```python
from build123d import *

# Parameters (mm, degrees)
SKETCH1_W            = 16.31
SKETCH1_H            = 16.31
SKETCH1_R            = 4.5
BOSS_EXTRUDE1_DEPTH  = 4
SKETCH3_R            = 1.5
CUT_EXTRUDE1_DEPTH   = 4
BOSS_EXTRUDE2_DEPTH  = 4
BOSS_EXTRUDE6_DEPTH  = 4
CUT_EXTRUDE3_DEPTH   = 4
BOSS_EXTRUDE7_DEPTH  = 4
BOSS_EXTRUDE9_DEPTH  = 4
SKETCH17_OUTSIDE_W   = 136.165
SKETCH17_OUTSIDE_H   = 117.232
CUT_EXTRUDE4_DEPTH   = 4
SKETCH18_R           = 1.5
BOSS_EXTRUDE10_DEPTH = 4
CUT_EXTRUDE5_DEPTH   = 4
SKETCH20_R           = 2
CUT_EXTRUDE6_DEPTH   = 10
SKETCH21_R           = 3
CUT_EXTRUDE7_DEPTH   = 2


with BuildPart() as part:
    # Sketch1 → Boss-Extrude1 (new body)
    with BuildSketch(Plane(origin=(0, 0, 0), x_dir=(1, 0, 0), z_dir=(0, 1, 0))):
        Rectangle(SKETCH1_W, SKETCH1_H)
        with Locations(Location((0, 0, 0), (0, 0, 270))):
            Circle(SKETCH1_R, mode=Mode.SUBTRACT)
    extrude(amount=BOSS_EXTRUDE1_DEPTH)

    # Sketch3 → Cut-Extrude1 (cut)
    with BuildSketch(Plane(origin=(0, 4, 0), x_dir=(1, 0, 0), z_dir=(0, 1, 0))):
        with Locations(Location((5.656854249, 5.656854249, 0), (0, 0, 270))):
            Circle(SKETCH3_R)
        with Locations(Location((5.656854249, -5.656854249, 0), (0, 0, 270))):
            Circle(SKETCH3_R)
        with Locations(Location((-5.656854249, -5.656854249, 0), (0, 0, 270))):
            Circle(SKETCH3_R)
        with Locations(Location((-5.656854249, 5.656854249, 0), (0, 0, 270))):
            Circle(SKETCH3_R)
    extrude(amount=-CUT_EXTRUDE1_DEPTH, mode=Mode.SUBTRACT)

    # Sketch4 → Boss-Extrude2 (add)
    with BuildSketch(Plane(origin=(0, 4, 0), x_dir=(1, 0, 0), z_dir=(0, 1, 0))):
        Polygon((8.155, -8.155), (0, -8.155), (0, -10.655), (10.655, -10.655), (10.655, 0), (8.155, 0), align=None)
    extrude(amount=-BOSS_EXTRUDE2_DEPTH)

    # Sketch9 → Boss-Extrude6 (add)
    with BuildSketch(Plane(origin=(0, 4, 0), x_dir=(1, 0, 0), z_dir=(0, 1, 0))):
        Polygon((71.061407011, -58.982568069), (7.593139788, -10.281653748), (10.613791504, -4.032054751), (84.193483815, -43.982568069), (90.501950314, -50.291034568), (96.061407011, -50.291034568), (96.061407011, -73.982568069), (81.061407011, -73.982568069), (81.061407011, -68.982568069), align=None)
    extrude(amount=-BOSS_EXTRUDE6_DEPTH)

    # Sketch12 → Cut-Extrude3 (cut)
    with BuildSketch(Plane(origin=(0, 4, 0), x_dir=(1, 0, 0), z_dir=(0, 1, 0))):
        Polygon((87.278639473, -47.258318902), (85.780514725, -48.583317861), (89.960889469, -52.761034568), (90.501950314, -52.761034568), (96.061407011, -52.761034568), (96.061407011, -50.291034568), (90.501950314, -50.291034568), (87.347717064, -47.136801318), align=None)
    extrude(amount=-CUT_EXTRUDE3_DEPTH, mode=Mode.SUBTRACT)

    # Sketch13 → Boss-Extrude7 (add)
    with BuildSketch(Plane(origin=(0, 4, 0), x_dir=(1, 0, 0), z_dir=(0, 1, 0))):
        Polygon((81.061407011, -73.982568069), (81.061407011, -77.282568069), (96.561407011, -77.282568069), (96.561407011, -52.761034568), (96.061407011, -52.761034568), (96.061407011, -73.982568069), align=None)
    extrude(amount=-BOSS_EXTRUDE7_DEPTH)

    # Sketch16 → Boss-Extrude9 (add)
    with BuildSketch(Plane(origin=(0, 4, 0), x_dir=(1, 0, 0), z_dir=(0, 1, 0))):
        Polygon((0, -10.655), (-10, -10.655), (-10, 10.345), (10.655, 10.345), (10.655, 0), (8.155, 0), (8.155, 8.155), (-8.155, 8.155), (-8.155, -8.155), (0, -8.155), align=None)
    extrude(amount=-BOSS_EXTRUDE9_DEPTH)

    # Sketch17 outside → Cut-Extrude4 (cut)
    with BuildSketch(Plane(origin=(0, 4, 0), x_dir=(1, 0, 0), z_dir=(0, 1, 0))):
        with Locations((43.2805, -33.469)):
            Rectangle(SKETCH17_OUTSIDE_W, SKETCH17_OUTSIDE_H)
        with BuildLine():
            Line((5.656854249, -8.656854249), (5.656854249, -10.655))
            Line((5.656854249, -10.655), (8.079694096, -10.655))
            Line((8.079694096, -10.655), (71.061407011, -58.982568069))
            Line((71.061407011, -58.982568069), (81.061407011, -68.982568069))
            Line((81.061407011, -68.982568069), (81.061407011, -77.282568069))
            Line((81.061407011, -77.282568069), (96.561407011, -77.282568069))
            Line((96.561407011, -77.282568069), (96.561407011, -52.761034568))
            Line((96.561407011, -52.761034568), (89.960889469, -52.761034568))
            Line((89.960889469, -52.761034568), (85.780514725, -48.583317861))
            Line((85.780514725, -48.583317861), (87.278639473, -47.258318902))
            Line((87.278639473, -47.258318902), (84.193483815, -43.982568069))
            Line((84.193483815, -43.982568069), (10.655, -4.054429139))
            Line((10.655, -4.054429139), (8.656854249, -5.656854249))
            ThreePointArc((8.656854249, -5.656854249), (6.313708499, 0), (8.656854249, 5.656854249))
            ThreePointArc((8.656854249, 5.656854249), (8.656854249, 8.656854249), (5.656854249, 8.656854249))
            ThreePointArc((5.656854249, 8.656854249), (0, 6.313708499), (-5.656854249, 8.656854249))
            ThreePointArc((-5.656854249, 8.656854249), (-8.656854249, 8.656854249), (-8.656854249, 5.656854249))
            ThreePointArc((-8.656854249, 5.656854249), (-6.313708499, 0), (-8.656854249, -5.656854249))
            ThreePointArc((-8.656854249, -5.656854249), (-8.656854249, -8.656854249), (-5.656854249, -8.656854249))
            ThreePointArc((-5.656854249, -8.656854249), (0, -6.313708499), (5.656854249, -8.656854249))
        make_face(mode=Mode.SUBTRACT)
    extrude(amount=-CUT_EXTRUDE4_DEPTH, mode=Mode.SUBTRACT)

    # Sketch18 → Boss-Extrude10 (add)
    with BuildSketch(Plane(origin=(0, 4, 0), x_dir=(1, 0, 0), z_dir=(0, 1, 0))):
        Polygon((5.656854249, -10.655), (0, -6.313708499), (6.372805828, -0.97060021), (10.655, -4.054429139), (8.656854249, -5.656854249), align=None)
        with Locations(Location((5.656854249, -5.656854249, 0), (0, 0, 270))):
            Circle(SKETCH18_R, mode=Mode.SUBTRACT)
    extrude(amount=-BOSS_EXTRUDE10_DEPTH)

    # Sketch19 → Cut-Extrude5 (cut)
    with BuildSketch(Plane(origin=(0, 4, 0), x_dir=(1, 0, 0), z_dir=(0, 1, 0))):
        with BuildLine():
            Line((97.061407011, -77.355955856), (97.061407011, -59.355955856))
            ThreePointArc((97.061407011, -59.355955856), (93.061407011, -61.012810105), (89.061407011, -59.355955856))
            ThreePointArc((89.061407011, -59.355955856), (92.789329073, -68.355955856), (89.061407011, -77.355955856))
            Line((89.061407011, -77.355955856), (97.061407011, -77.355955856))
        make_face()
    extrude(amount=-CUT_EXTRUDE5_DEPTH, mode=Mode.SUBTRACT)

    # Sketch20 → Cut-Extrude6 (cut)
    with BuildSketch(Plane.XZ):
        with Locations(Location((81.807805677, 62.103797793, 0), (0, 0, 270))):
            Circle(SKETCH20_R)
    extrude(amount=-CUT_EXTRUDE6_DEPTH, mode=Mode.SUBTRACT)

    # Sketch21 → Cut-Extrude7 (cut)
    with BuildSketch(Plane.XZ):
        with Locations(Location((81.807805677, 62.103797793, 0), (0, 0, 270))):
            Circle(SKETCH21_R)
    extrude(amount=-CUT_EXTRUDE7_DEPTH, mode=Mode.SUBTRACT)


solid = part.part
```
Build history of the part. All positions in model axes, mm. A direction names the side the tool comes from. Round coordinates to 2 decimals unless told otherwise and drop trailing zeros. Loops run counter-clockwise (first coordinate to the right, second up) from the corner with the lowest first, then second, coordinate; pieces in that order, holes last.
Item 1: Drill centre lines: line 1 along Z through (x, y) = (-5, 0.4); line 2 along X through (y, z) = (1, 62.5); line 3 along X through (y, z) = (2.4, 30). Where is each one in solid material? Low to high.
Item 2: Pin check, flat tips, straight feed: P1, Ø3, axis at x = 81.81, z = 62.1, coming from the -Y side; P2, Ø1.9, axis at x = 6.5, y = 2.5, coming from the +Z side (3 decimals); P3, Ø1.2, axis at y = 2, z = 72, coming from the -X side; P4, Ø1.5, axis at y = 0.5, z = 32.5, coming from the -X side. Stop position of each tip, or through.
Item 3: Saw through at B-B (x = 65). List the corners of the cut face in (y, z).
Item 4: Two-plate mould, pull along X, no slides. Class faces 4 (the face through (93, 2, 52.761)), 5 (the face through (46.91, 2.03, 23.74)), 6 (the face through (-6.314, 2.028, -0.088)), 7 (the face through (-3.1, 2.03, 6.94)): released by +X, released by -X, zero draft, split by the parting line, or undercut.
Item 5: Saw through at A-A (y = 3.1). List the corners of the cut face in (x, z) (3 decimals).
Item 6: Saw through at C-C (z = 35.5). List the corners of the cut face in (x, y).
Item 7: Which spindle directions (+Z, -Z, +X, -X, +Y, -Y) get a long thin tool onto all of the face, cutting with end or side? Do faces 1 (the face through (7, 2, 10.655)), 2 (the face through (87.8, 2, 50.6)), 3 (the face through (80, 1, 64.5)). Say none if no direction does.
Worked answers:
1. line 1: z = -8.07 to -7.01, -4.31 to 4.31, 7.01 to 8.07
1. line 2: x = 74.58 to 78.83, 84.78 to 91.36
1. line 3: x = 33.29 to 58.44
2. P1: passes through
2. P2: stops at z = 10.655
2. P3: stops at x = 81.06
2. P4: stops at x = 35.57
3. outline: (0, 33.56) - (4, 33.56) - (4, 54.33) - (0, 54.33) - close
4. face 4: zero draft
4. face 5: released by +X
4. face 6: released by -X
4. face 7: undercut
5. outline: (-8.657, -5.657) arc R2.121 ccw to (-5.657, -8.657) arc R8 cw to (5.657, -8.657) arc R2.121 ccw to (8.657, -5.657) arc R8 cw to (6.373, 0.971) - (10.655, 4.054) - (84.193, 43.983) - (87.279, 47.258) - (85.781, 48.583) - (89.961, 52.761) - (96.561, 52.761) - (96.561, 59.8) arc R5.657 ccw to (89.061, 59.356) arc R12.728 ccw to (89.134, 77.283) - (81.061, 77.283) - (81.061, 68.983) - (71.061, 58.983) - (8.08, 10.655) - (5.657, 10.655) - (0, 6.314) arc R8 cw to (-5.657, 8.657) arc R2.121 ccw to (-8.657, 5.657) arc R8 cw to start; hole circle Ø3 at (-5.657, -5.657); hole circle Ø3 at (-5.657, 5.657); hole circle Ø9 at (0, 0); hole circle Ø3 at (5.657, -5.657); hole circle Ø3 at (5.657, 5.657); hole circle Ø4 at (81.808, 62.104)
6. outline: (40.46, 0) - (68.57, 0) - (68.57, 4) - (40.46, 4) - close
7. face 1: +Z, -X, +Y, -Y
7. face 2: +X, +Y, -Y
7. face 3: -Y
